```python
from build123d import *

# Parameters (mm, degrees)
BOSS_EXTRUDE2_DEPTH = 100
CUT_EXTRUDE1_DEPTH  = 30


with BuildPart() as part:
    # Sketch2 → Boss-Extrude2 (new body)
    with BuildSketch(Plane(origin=(0, 0, 0), x_dir=(1, 0, 0), z_dir=(0, 1, 0))):
        with BuildLine():
            Line((-15, -5), (15, -5))
            ThreePointArc((15, -5), (20, 0), (15, 5))
            Line((15, 5), (-15, 5))
            ThreePointArc((-15, 5), (-20, 0), (-15, -5))
        make_face()
    extrude(amount=BOSS_EXTRUDE2_DEPTH)

    # Sketch3 → Cut-Extrude1 (cut)
    with BuildSketch(Plane(origin=(0, 0, 0), x_dir=(-1, 0, 0), z_dir=(0, -1, 0))):
        with BuildLine():
            ThreePointArc((2.55, 0), (1.803122292, 1.803122292), (0, 2.55))
            Line((0, 2.55), (0, -2.55))
            ThreePointArc((0, -2.55), (1.803122292, -1.803122292), (2.55, 0))
        make_face()
        with BuildLine():
            Line((0, -2.55), (0, 2.55))
            ThreePointArc((0, 2.55), (-2.55, 0), (0, -2.55))
        make_face()
    extrude(amount=-CUT_EXTRUDE1_DEPTH, mode=Mode.SUBTRACT)


solid = part.part
```
CAD build for the part. Positions are in the model's coordinates, mm. Coordinates: 2 decimals unless noted, no trailing zeros. Order: outer loops, then holes, each group sorted by start corner. A loop starts at its lowest first (then second) coordinate and runs counter-clockwise, first axis right, second up. Notation, with made-up numbers: (15, 64.5) - (73, 64.5) arc R29 cw to (73, 88.5) - close; hole circle Ø4 at (1, 8). An arc over 180 degrees is marked (long way). Use a Markdown table: item, result. Add a question column.
(1) Saw through at D-D (z = 3.5). Give the cut face in (x, y).
(2) Pull direction X, two halves, no side cores. Call faces 1 (the face through (0, 30, 0)), 2 (the face through (0, 49, 5)), 3 (the face through (20, 49, 0)), 4 (the face through (-20, 49, 0)): +X half, -X half, draft (parallel to the pull), parting line (faces both ways), or undercut.
(3) Drill centre lines: line 1 along X through (y, z) = (4, 0); line 2 along Z through (x, y) = (-2, 23); line 3 along X through (y, z) = (27, 4). Where is each one in solid material? Low to high. Write a range as [from, to].
(4) Flat gauge pin, fed straight in: pin 1 (1.5 mm diameter, centred on x = 1, z = 0, fed in from -Y). Where does the tip first touch, or does it go through?
(5) Saw through at C-C (x = -1.5). Give the cut face in (y, z).
(6) Saw through at A-A (y = 11.5). Give the cut face in (x, z), then the cut area to 3 significant figures.
(7) Saw through at B-B (y = 68). Give the cut face in (x, z).
Solved:
| question | item | result |
|---|---|---|
| 1 | outline | (-18.57, 0) - (18.57, 0) - (18.57, 100) - (-18.57, 100) - close |
| 2 | face 1 | undercut |
| 2 | face 2 | draft |
| 2 | face 3 | +X half |
| 2 | face 4 | -X half |
| 3 | line 1 | x = [-20, -2.55], [2.55, 20] |
| 3 | line 2 | z = [-5, -1.58], [1.58, 5] |
| 3 | line 3 | x = [-18, 18] |
| 4 | pin 1 | stops at y = 30 |
| 5 | outline | (0, -5) - (100, -5) - (100, 5) - (0, 5) - (0, 2.06) - (30, 2.06) - (30, -2.06) - (0, -2.06) - close |
| 6 | outline | (-15, -5) - (15, -5) arc R5 ccw to (15, 5) - (-15, 5) arc R5 ccw to start; hole circle Ø5.1 at (0, 0) |
| 6 | area | 358 mm² |
| 7 | outline | (-15, -5) - (15, -5) arc R5 ccw to (15, 5) - (-15, 5) arc R5 ccw to start |
